Here's how the part is built. I have some questions about the finished solid (model axes, mm). A direction names the side the tool comes from. Coordinates: 2 decimals unless noted, no trailing zeros. Loops run counter-clockwise (first coordinate to the right, second up) from the corner with the lowest first, then second, coordinate; pieces in that order, holes last.
from build123d import *

# Parameters (mm, degrees)
BOSS_EXTRUDE1_DEPTH = 6.5
BOSS_EXTRUDE2_DEPTH = 1.2


with BuildPart() as part:
    # Sketch1 → Boss-Extrude1 (new body)
    with BuildSketch(Plane.XY):
        with BuildLine():
            Line((-54.735153148, 20.85842627), (-54.735153148, 20.05842627))
            ThreePointArc((-54.735153148, 20.05842627), (-53.835153148, 19.15842627), (-52.935153148, 20.05842627))
            Line((-52.935153148, 20.05842627), (-52.935153148, 20.85842627))
            ThreePointArc((-52.935153148, 20.85842627), (-53.835153148, 21.75842627), (-54.735153148, 20.85842627))
        make_face()
    extrude(amount=BOSS_EXTRUDE1_DEPTH)

    # Sketch3 → Boss-Extrude2 (add)
    with BuildSketch(Plane(origin=(0, 0, 0), x_dir=(-1, 0, 0), z_dir=(0, 0, -1))):
        with BuildLine():
            Line((51.935153148, 20.85842627), (51.935153148, 16.05842627))
            Line((51.935153148, 16.05842627), (55.735153148, 16.05842627))
            Line((55.735153148, 16.05842627), (55.735153148, 20.85842627))
            ThreePointArc((55.735153148, 20.85842627), (53.835153148, 22.75842627), (51.935153148, 20.85842627))
        make_face()
    extrude(amount=BOSS_EXTRUDE2_DEPTH)


solid = part.part
Q1. Suppose I cut it at C-C on z = 1.5. Write out the boundary of the cut face in (x, y).
Q2. Will this pin go through, and if not, where does the flat tip stop? P1, Ø0.9, axis at y = 20.5, z = 4, coming from the +X side.
Q3. For faces 1 (the flat face through (-52.935, 20.5, 3.2)), 2 (the cylindrical face through (-53.85, 19.16, 3.2)), 3 (the flat face through (-54, 19, 0)), 4 (the cylindrical face through (-53.82, 21.76, 3.2)), 5 (the flat face through (-54.735, 20.5, 3.2)), which set-ups out of +Z, -Z, +X, -X, +Y, -Y let a thin tool reach every point of the face, with its end or its side?
Q4. Suppose I cut it at D-D on y = 19. Write out the boundary of the cut face in (x, z), and give its area (3 significant figures).
Q5. Suppose I cut it at B-B on x = -53.4. Write out the boundary of the cut face in (y, z).
Q6. Please list where these lines run through material, in increasing order: probe 1 along X at (y, z) = (20, 2.5); probe 2 along Z at (x, y) = (-52.2, 20.75); probe 3 along Y at (x, z) = (-53.85, 5.75).
Q7. Suppose I cut it at A-A on y = 20.75. Write out the boundary of the cut face in (x, z), and give its area (3 significant figures).
Check values:
1. outline: (-54.74, 20.06) arc R0.9 ccw to (-52.94, 20.06) - (-52.94, 20.86) arc R0.9 ccw to (-54.74, 20.86) - close
2. P1: stops at x = -52.94
3. face 1: +Z, +X, +Y, -Y
3. face 2: +Z, -Y
3. face 3: +Z
3. face 4: +Z, +Y
3. face 5: +Z, -X, +Y, -Y
4. outline: (-55.74, -1.2) - (-51.94, -1.2) - (-51.94, 0) - (-55.74, 0) - close
4. area: 4.56 mm2
5. outline: (16.06, -1.2) - (22.71, -1.2) - (22.71, 0) - (21.65, 0) - (21.65, 6.5) - (19.27, 6.5) - (19.27, 0) - (16.06, 0) - close
6. probe 1: x = -54.73 to -52.94
6. probe 2: z = -1.2 to 0
6. probe 3: y = 19.16 to 21.76
7. outline: (-55.74, -1.2) - (-51.94, -1.2) - (-51.94, 0) - (-52.94, 0) - (-52.94, 6.5) - (-54.74, 6.5) - (-54.74, 0) - (-55.74, 0) - close
7. area: 16.3 mm2
